Autodesk Inventor part; units mm, degrees
ref_plane "YZ Plane" through (0, 0, 0) normal (1, 0, 0) x (0, 1, 0)
ref_plane "XZ Plane" through (0, 0, 0) normal (0, 1, 0) x (-1, 0, 0)
ref_plane "XY Plane" through (0, 0, 0) normal (0, 0, 1) x (1, 0, 0)
sketch "Sketch1" plane through (0, 0, 0) normal (0, 0, 1) x (1, 0, 0)
  circle A0 centre (-16, 0) radius 2.75
  circle A1 centre (16, 0) radius 2.75
  circle A2 centre (0, 0) radius 4
  circle A3 centre (-16, 0) radius 5.25
  circle A4 centre (16, 0) radius 5.25
  circle A5 centre (0, 0) radius 10
  line L0 (-2.9687, 9.5492) -> (-17.5586, 5.0133)
  line L1 (2.9687, 9.5492) -> (17.5586, 5.0133)
  line L2 (-17.5586, -5.0133) -> (-2.9688, -9.5492)
  line L3 (2.9687, -9.5492) -> (17.5586, -5.0133)
  line L4 (-10, 3.0548) -> (10, 3.0548)
  line L5 (10, 3.0548) -> (10, -14)
  line L6 (10, -14) -> (-10, -14)
  line L7 (-10, -14) -> (-10, 3.0548)
  line L8 (-0.75, 0) -> (0.75, 0)
  line L9 (0.75, 0) -> (0.75, -14)
  line L10 (0.75, -14) -> (-0.75, -14)
  line L11 (-0.75, -14) -> (-0.75, 0)
  point P0 (-9.522, 3.0548)
  point P1 (-10, 0)
  point P2 (-10, -7.3632)
  point P3 (-0.75, -3.9291)
  point P4 (0.75, -3.9291)
  point P5 (10, -7.3632)
  point P6 (9.522, 3.0548)
  point P7 (10, 0)
  dimension "d0" = 5.5
  dimension "d1" = 5.5
  dimension "d2" = 32
  dimension "d3" = 16
  dimension "d4" = 8
  dimension "d5" = 10.5
  dimension "d6" = 10.5
  dimension "d7" = 20
  dimension "d8" = 0
  dimension "d9" = 0
  dimension "d10" = 14
  dimension "d11" = 20
  dimension "d12" = 10
  dimension "d13" = 1.5
  dimension "d14" = 0.75
extrude "Extrusion1" add sketch "Sketch1" along normal blind 10 contours A2 L4 A5 L9 | A2 L4 A5 | A2 L11 A5 L4 | L4 L5 A5 | A5 L1 A4 L3 L5 L4 | A5 L3 L5 L6 L9 | L4 L7 L2 A3 L0 A5 | A5 L7 L4 | L5 L3 A5 | L11 L6 L7 L2 A5 | A5 L2 L7 | A4 | A3
properties part number "SHF08"
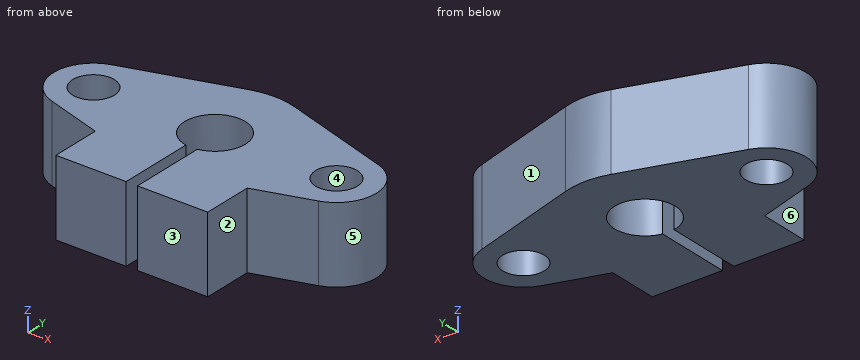
Geometry: final body of the model. Coordinates: model frame, mm. Face numbers are marked on the shaded views. A direction names the side the tool comes from. Round coordinates to 2 decimals unless told otherwise and drop trailing zeros. Write each loop counter-clockwise with the first axis right and the second up, starting at its lowest first coordinate (ties: lowest second). Pieces come first, ordered by that corner, then holes.
Item 1: Section query B-B (z = 5.25). Return loops of the section in (x, y).
Item 2: Mould query, pull axis Y, two halves, no side actions, for the marked faces 1, 2, 3 and 4. Classes: +Y half, -Y half, draft (parallel to the pull), parting line (faces both ways), or undercut.
Item 3: Material intervals for L1, parallel to X at y = -10, z = 3.5; L2, parallel to X at y = -2.5, z = 6.5; L3, parallel to Y at x = 0, z = 4.5, sorted ascending.
Item 4: Pin query (flat end, axial travel): P1, Ø12, axis at x = 16.5, y = 5.5, coming from the -Z side; P2, Ø2, axis at y = -12, z = 6, coming from the +X side; P3, Ø7, axis at x = 0, y = 0, coming from the -Z side. Return the tip coordinate at first contact, or that it passes through.
Item 5: Section query D-D (x = 16). Return loops of the section in (y, z), plus the area to 3 significant figures.
Item 6: Set-up query: the marked faces 5 and 6. Return all of +Z, -Z, +X, -X, +Y, -Y with unobstructed straight access to the full face (end or side cutting, diameter ignored); none if empty.
Item 7: Section query A-A (y = -9.5). Return loops of the section in (x, z), plus the area to 3 significant figures.
Item 8: Section query C-C (y = 0). Return loops of the section in (x, z), plus the area to 3 significant figures.
Completed:
1. outline: (-17.56, -5.01) - (-10, -7.36) - (-10, -14) - (-0.75, -14) - (-0.75, -3.93) arc R4 cw (long way) to (0.75, -3.93) - (0.75, -14) - (10, -14) - (10, -7.36) - (17.56, -5.01) arc R5.25 ccw to (17.56, 5.01) - (2.97, 9.55) arc R10 ccw to (-2.97, 9.55) - (-17.56, 5.01) arc R5.25 ccw to start; hole circle Ø5.5 at (-16, 0); hole circle Ø5.5 at (16, 0)
2. face 1: +Y half
2. face 2: draft
2. face 3: -Y half
2. face 4: undercut
3. L1: x = -10 to -0.75, 0.75 to 10
3. L2: x = -20.62 to -17.15, -14.85 to -3.12, 3.12 to 14.85, 17.15 to 20.62
3. L3: y = 4 to 10
4. P1: stops at z = 0
4. P2: stops at x = 10
4. P3: passes through
5. outline: (-5.5, 0) - (-2.75, 0) - (-2.75, 10) - (-5.5, 10) - close; (2.75, 0) - (5.5, 0) - (5.5, 10) - (2.75, 10) - close
5. area: 55.0 mm2
6. face 5: +Z, -Z, +X
6. face 6: +Z, -Z, -X, -Y
7. outline: (-10, 0) - (-0.75, 0) - (-0.75, 10) - (-10, 10) - close; (0.75, 0) - (10, 0) - (10, 10) - (0.75, 10) - close
7. area: 185 mm2
8. outline: (-21.25, 0) - (-18.75, 0) - (-18.75, 10) - (-21.25, 10) - close; (-13.25, 0) - (-4, 0) - (-4, 10) - (-13.25, 10) - close; (4, 0) - (13.25, 0) - (13.25, 10) - (4, 10) - close; (18.75, 0) - (21.25, 0) - (21.25, 10) - (18.75, 10) - close
8. area: 235 mm2
